from build123d import *

# Parameters (mm, degrees)
SKETCH1_W                  = 10
SKETCH1_H                  = 7
CUT_EXTRUDE1_DEPTH         = 25.841675415
CUT_EXTRUDE2_DEPTH         = 25.841675415
CUT_EXTRUDE3_DEPTH         = 25.841675415
CUT_EXTRUDE4_DEPTH         = 25.841675415
CUT_EXTRUDE5_DEPTH         = 25.841675415
CUT_EXTRUDE6_DEPTH         = 25.841675415
CUT_EXTRUDE7_DEPTH         = 25.841675415
CUT_EXTRUDE8_DEPTH         = 25.841675415
CUT_EXTRUDE9_DEPTH         = 25.73038126
CUT_EXTRUDE10_DEPTH        = 25.73038126
CUT_EXTRUDE11_DEPTH        = 25.73038126
CUT_EXTRUDE12_DEPTH        = 25.590210189
SKETCH14_W                 = 30.0000508
SKETCH14_H                 = 2.5
F_0_8_0_8_DIAMETER_HOLE1_D = 0.8
BOSS_EXTRUDE1_START        = -40.0000508
SKETCH17_R                 = 0.4
BOSS_EXTRUDE1_DEPTH        = 40.0000508
SKETCH18_W                 = 1.5
SKETCH18_H                 = 1.5
CHAMFER1_SIZE              = 0.5
CUT_EXTRUDE13_REACH        = 34.638
CUT_EXTRUDE13_END_RADIUS   = 2
CUT_EXTRUDE13_START        = 5
FILLET1_R                  = 0.5


# Read off the part's stored shape, not the designer's step: Dome1
with BuildPart() as part:
    # Sketch1 → Revolve1 (revolve)
    with BuildSketch(Plane(origin=(0, 0, -7.196357143), x_dir=(-1, 0, 0), z_dir=(0, 0, -1)), mode=Mode.PRIVATE) as revolve1_sk:
        with Locations((-14.77870785, 14.264354232)):
            Rectangle(SKETCH1_W, SKETCH1_H)
    revolve(revolve1_sk.sketch.rotate(Axis((19.77870785, 10.764354232, -7.196357143), (-1, 0, 0)), 270), axis=Axis((19.77870785, 10.764354232, -7.196357143), (-1, 0, 0)))

    # Sketch2 → Cut-Extrude1 (cut, through all)
    with BuildSketch(Plane.ZY.offset(-9.77870785)):
        with BuildLine():
            ThreePointArc((-0.481894482, 12.743240579), (-1.134179317, 14.264354232), (-2.125359964, 15.589806295))
            ThreePointArc((-2.125359964, 15.589806295), (-2.500220073, 14.433413298), (-3.393627672, 13.609042188))
            ThreePointArc((-3.393627672, 13.609042188), (-3.083602501, 13.138854232), (-2.831420372, 12.635270579))
            ThreePointArc((-2.831420372, 12.635270579), (-1.670790249, 12.996798701), (-0.481894482, 12.743240579))
        make_face()
    extrude(amount=-CUT_EXTRUDE1_DEPTH, mode=Mode.SUBTRACT)

    # Sketch3 → Cut-Extrude2 (cut, through all)
    with BuildSketch(Plane.ZY.offset(-9.77870785)):
        with BuildLine():
            ThreePointArc((-0.392018732, 9.12088875), (-0.196357143, 10.764354232), (-0.392018732, 12.407819713))
            ThreePointArc((-0.392018732, 12.407819713), (-1.294853608, 11.593784056), (-2.480752839, 11.326561532))
            ThreePointArc((-2.480752839, 11.326561532), (-2.447357143, 10.764354232), (-2.480752839, 10.202146931))
            ThreePointArc((-2.480752839, 10.202146931), (-1.294853608, 9.934924408), (-0.392018732, 9.12088875))
        make_face()
    extrude(amount=-CUT_EXTRUDE2_DEPTH, mode=Mode.SUBTRACT)

    # Sketch4 → Cut-Extrude3 (cut, through all)
    with BuildSketch(Plane.ZY.offset(-9.77870785)):
        with BuildLine():
            ThreePointArc((-2.125359964, 5.938902169), (-1.134179317, 7.264354232), (-0.481894482, 8.785467884))
            ThreePointArc((-0.481894482, 8.785467884), (-1.670790249, 8.531909762), (-2.831420372, 8.893437884))
            ThreePointArc((-2.831420372, 8.893437884), (-3.083602501, 8.389854232), (-3.393627672, 7.919666275))
            ThreePointArc((-3.393627672, 7.919666275), (-2.500220073, 7.095295166), (-2.125359964, 5.938902169))
        make_face()
    extrude(amount=-CUT_EXTRUDE3_DEPTH, mode=Mode.SUBTRACT)

    # Sketch5 → Cut-Extrude4 (cut, through all)
    with BuildSketch(Plane.ZY.offset(-9.77870785)):
        with BuildLine():
            ThreePointArc((-5.217470795, 4.049891571), (-3.696357143, 4.702176405), (-2.37090508, 5.693357053))
            ThreePointArc((-2.37090508, 5.693357053), (-3.527298077, 6.068217161), (-4.351669187, 6.96162476))
            ThreePointArc((-4.351669187, 6.96162476), (-4.821857143, 6.651599589), (-5.325440796, 6.39941746))
            ThreePointArc((-5.325440796, 6.39941746), (-4.963912674, 5.238787337), (-5.217470795, 4.049891571))
        make_face()
    extrude(amount=-CUT_EXTRUDE4_DEPTH, mode=Mode.SUBTRACT)

    # Sketch6 → Cut-Extrude5 (cut, through all)
    with BuildSketch(Plane.ZY.offset(-9.77870785)):
        with BuildLine():
            ThreePointArc((-8.839822625, 3.960015821), (-7.196357143, 3.764354232), (-5.552891661, 3.960015821))
            ThreePointArc((-5.552891661, 3.960015821), (-6.366927319, 4.862850696), (-6.634149843, 6.048749928))
            ThreePointArc((-6.634149843, 6.048749928), (-7.196357143, 6.015354232), (-7.758564444, 6.048749928))
            ThreePointArc((-7.758564444, 6.048749928), (-8.025786967, 4.862850696), (-8.839822625, 3.960015821))
        make_face()
    extrude(amount=-CUT_EXTRUDE5_DEPTH, mode=Mode.SUBTRACT)

    # Sketch7 → Cut-Extrude6 (cut, through all)
    with BuildSketch(Plane.ZY.offset(-9.77870785)):
        with BuildLine():
            ThreePointArc((-12.021809206, 5.693357053), (-10.696357143, 4.702176405), (-9.175243491, 4.049891571))
            ThreePointArc((-9.175243491, 4.049891571), (-9.428801613, 5.238787337), (-9.067273491, 6.39941746))
            ThreePointArc((-9.067273491, 6.39941746), (-9.570857143, 6.651599589), (-10.0410451, 6.96162476))
            ThreePointArc((-10.0410451, 6.96162476), (-10.865416209, 6.068217161), (-12.021809206, 5.693357053))
        make_face()
    extrude(amount=-CUT_EXTRUDE6_DEPTH, mode=Mode.SUBTRACT)

    # Sketch8 → Cut-Extrude7 (cut, through all)
    with BuildSketch(Plane.ZY.offset(-9.77870785)):
        with BuildLine():
            ThreePointArc((-13.910819804, 8.785467884), (-13.25853497, 7.264354232), (-12.267354322, 5.938902169))
            ThreePointArc((-12.267354322, 5.938902169), (-11.892494213, 7.095295166), (-10.999086614, 7.919666275))
            ThreePointArc((-10.999086614, 7.919666275), (-11.309111786, 8.389854232), (-11.561293915, 8.893437884))
            ThreePointArc((-11.561293915, 8.893437884), (-12.721924037, 8.531909762), (-13.910819804, 8.785467884))
        make_face()
    extrude(amount=-CUT_EXTRUDE7_DEPTH, mode=Mode.SUBTRACT)

    # Sketch9 → Cut-Extrude8 (cut, through all)
    with BuildSketch(Plane.ZY.offset(-9.77870785)):
        with BuildLine():
            ThreePointArc((-14.000695554, 12.407819713), (-14.196357143, 10.764354232), (-14.000695554, 9.12088875))
            ThreePointArc((-14.000695554, 9.12088875), (-13.097860679, 9.934924408), (-11.911961447, 10.202146931))
            ThreePointArc((-11.911961447, 10.202146931), (-11.945357143, 10.764354232), (-11.911961447, 11.326561532))
            ThreePointArc((-11.911961447, 11.326561532), (-13.097860679, 11.593784056), (-14.000695554, 12.407819713))
        make_face()
    extrude(amount=-CUT_EXTRUDE8_DEPTH, mode=Mode.SUBTRACT)

    # Sketch10 → Cut-Extrude9 (cut, through all)
    with BuildSketch(Plane.ZY.offset(-9.77870785)):
        with BuildLine():
            ThreePointArc((-12.267354322, 15.589806295), (-13.25853497, 14.264354232), (-13.910819804, 12.743240579))
            ThreePointArc((-13.910819804, 12.743240579), (-12.721924037, 12.996798701), (-11.561293915, 12.635270579))
            ThreePointArc((-11.561293915, 12.635270579), (-11.309111786, 13.138854232), (-10.999086614, 13.609042188))
            ThreePointArc((-10.999086614, 13.609042188), (-11.892494213, 14.433413298), (-12.267354322, 15.589806295))
        make_face()
    extrude(amount=-CUT_EXTRUDE9_DEPTH, mode=Mode.SUBTRACT)

    # Sketch11 → Cut-Extrude10 (cut, through all)
    with BuildSketch(Plane.ZY.offset(-9.77870785)):
        with BuildLine():
            ThreePointArc((-9.175243491, 17.478816892), (-10.696357143, 16.826532058), (-12.021809206, 15.83535141))
            ThreePointArc((-12.021809206, 15.83535141), (-10.865416209, 15.460491302), (-10.0410451, 14.567083703))
            ThreePointArc((-10.0410451, 14.567083703), (-9.570857143, 14.877108874), (-9.067273491, 15.129291003))
            ThreePointArc((-9.067273491, 15.129291003), (-9.428801613, 16.289921126), (-9.175243491, 17.478816892))
        make_face()
    extrude(amount=-CUT_EXTRUDE10_DEPTH, mode=Mode.SUBTRACT)

    # Sketch12 → Cut-Extrude11 (cut, through all)
    with BuildSketch(Plane.ZY.offset(-9.77870785)):
        with BuildLine():
            ThreePointArc((-5.552891661, 17.568692642), (-7.196357143, 17.764354232), (-8.839822625, 17.568692642))
            ThreePointArc((-8.839822625, 17.568692642), (-8.025786967, 16.665857767), (-7.758564444, 15.479958536))
            ThreePointArc((-7.758564444, 15.479958536), (-7.196357143, 15.513354232), (-6.634149843, 15.479958536))
            ThreePointArc((-6.634149843, 15.479958536), (-6.366927319, 16.665857767), (-5.552891661, 17.568692642))
        make_face()
    extrude(amount=-CUT_EXTRUDE11_DEPTH, mode=Mode.SUBTRACT)

    # Sketch13 → Cut-Extrude12 (cut, through all)
    with BuildSketch(Plane.ZY.offset(-9.77870785)):
        with BuildLine():
            ThreePointArc((-2.37090508, 15.83535141), (-3.696357143, 16.826532058), (-5.217470795, 17.478816892))
            ThreePointArc((-5.217470795, 17.478816892), (-4.963912674, 16.289921126), (-5.325440796, 15.129291003))
            ThreePointArc((-5.325440796, 15.129291003), (-4.821857143, 14.877108874), (-4.351669187, 14.567083703))
            ThreePointArc((-4.351669187, 14.567083703), (-3.527298077, 15.460491302), (-2.37090508, 15.83535141))
        make_face()
    extrude(amount=-CUT_EXTRUDE12_DEPTH, mode=Mode.SUBTRACT)

    # Sketch14 → Revolve2 (revolve)
    with BuildSketch(Plane.XY.offset(-7.196357143), mode=Mode.PRIVATE) as revolve2_sk:
        with Locations((-5.22131755, 12.014354232)):
            Rectangle(SKETCH14_W, SKETCH14_H)
    revolve(revolve2_sk.sketch.rotate(Axis((-20.22134295, 10.764354232, -7.196357143), (1, 0, 0)), 270), axis=Axis((-20.22134295, 10.764354232, -7.196357143), (1, 0, 0)))

    # Ø0.8 (0.8) Diameter Hole1 (through all)
    with Locations(Plane(origin=(19.77870785, 0, 0), x_dir=(0, 0, -1), z_dir=(1, 0, 0))):
        with Locations((7.196357143, 10.764354232)):
            Hole(F_0_8_0_8_DIAMETER_HOLE1_D / 2)

    # Sketch17 → Boss-Extrude1 (add)
    with BuildSketch(Plane(origin=(19.77870785, 0, 0), x_dir=(0, 0, -1), z_dir=(1, 0, 0)).offset(BOSS_EXTRUDE1_START)):
        with Locations((7.196357143, 10.764354232)):
            Circle(SKETCH17_R)
    extrude(amount=BOSS_EXTRUDE1_DEPTH)

    # Sketch18 → Revolve3 (revolve)
    with BuildSketch(Plane.XY.offset(-7.196357143), mode=Mode.PRIVATE) as revolve3_sk:
        with Locations((-9.47134295, 14.014354232)):
            Rectangle(SKETCH18_W, SKETCH18_H)
    revolve(revolve3_sk.sketch.rotate(Axis((-20.22134295, 10.764354232, -7.196357143), (1, 0, 0)), 90), axis=Axis((-20.22134295, 10.764354232, -7.196357143), (1, 0, 0)))

    # Chamfer1
    chamfer1_edges = [part.edges().sort_by_distance(p)[0] for p in [
        (-20.22134295, 10.764354232, -4.696357143),
    ]]
    chamfer(chamfer1_edges, length=CHAMFER1_SIZE)

    # Cut-Extrude13: up to this cylinder (the profile starts outside it)
    cut_extrude13_end = Plane(origin=(-15.221343, 10.764354232, -7.196357143), z_dir=(1, 0, 0)) * Cylinder(CUT_EXTRUDE13_END_RADIUS, 74.276, mode=Mode.PRIVATE)
    # Sketch20 → Cut-Extrude13 (cut, up to the surface)
    with BuildSketch(Plane.XY.offset(-7.196357143).offset(CUT_EXTRUDE13_START), mode=Mode.PRIVATE) as cut_extrude13_sk1:
        with BuildLine():
            Line((-12.72134295, 9.882388481), (-17.72134295, 9.882388481))
            ThreePointArc((-17.72134295, 9.882388481), (-18.47134295, 10.632388481), (-17.72134295, 11.382388481))
            Line((-17.72134295, 11.382388481), (-12.72134295, 11.382388481))
            ThreePointArc((-12.72134295, 11.382388481), (-11.97134295, 10.632388481), (-12.72134295, 9.882388481))
        make_face()
    cut_extrude13_tool1 = extrude(cut_extrude13_sk1.sketch, amount=-CUT_EXTRUDE13_REACH, mode=Mode.PRIVATE) - cut_extrude13_end
    add(cut_extrude13_tool1.solids().sort_by_distance((-15.221343, 10.632388, -2.196357))[0], mode=Mode.SUBTRACT)

    # Dome1 outline → Dome1 (revolve, cut)
    with BuildSketch(Plane(origin=(0, 10.764354232, -7.196357143), x_dir=(0, 1, 0), z_dir=(0, 0, -1))):
        with BuildLine():
            Line((0, 19.778707854), (0, 19.27870785))
            ThreePointArc((0, 19.27870785), (1.891593251, 19.404258523), (3.750000014, 19.778707854))
            Line((3.750000014, 19.778707854), (0, 19.778707854))
        make_face()
    revolve(axis=Axis((0, 10.764354232, -7.196357143), (1, 0, 0)), mode=Mode.SUBTRACT)

    # Fillet1
    fillet1_edges = [part.edges().sort_by_distance(p)[0] for p in [
        (19.778707854, 7.014354218, -7.196357143),
    ]]
    fillet(fillet1_edges, radius=FILLET1_R)


solid = part.part
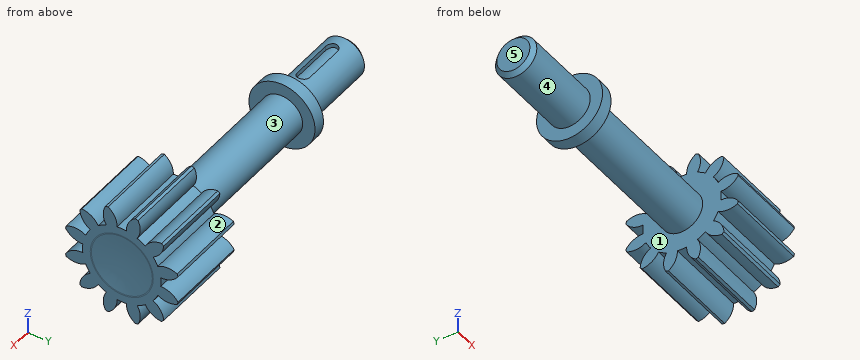
Source: CAD feature listing. Evaluate the final solid. Frame: model axes, mm. Face numbers are marked on the shaded views. A direction names the side the tool comes from. Round coordinates to 2 decimals unless told otherwise and drop trailing zeros. Loops run counter-clockwise (first coordinate to the right, second up) from the corner with the lowest first, then second, coordinate; pieces in that order, holes last. Notation, with made-up numbers: (15, 58) -> (33, 58) arc R15 ccw to (33, 63) -> close; hole circle Ø9 at (9.25, 23.25). An arc over 180 degrees is marked (long way). Answer as a JSON object with one key per item and string values. Group by question number.
Q1. Section query B-B (y = 16.5). Output: boundary loops of the cut face in (x, z), plus the area to 3 significant figures.
Q2. Access query for the marked faces 4 and 5. Directions: +Z, -Z, +X, -X, +Y, -Y. A direction counts if a zero-diameter tool reaches every point of the face in a straight line with its end or side. Return the directions, or none.
Q3. Section query C-C (x = 1). Output: boundary loops of the cut face in (y, z).
Q4. Mould query, pull axis Y, two halves, no side actions, for the marked faces 1, 2 and 3. Classes: pulls with the +Y half, pulls with the -Y half, needs draft (parallel to the pull), parting line crosses it, or undercut.
Q5. Ray query, line 1 (X direction, y = 14.25, z = -8.75); line 2 (X direction, y = 5, z = -8.5); line 3 (X direction, y = 8.75, z = -9.5). Return the intervals inside material, ascending. Write a range as from..to.
Q6. Section query A-A (y = 5.25). Output: boundary loops of the cut face in (x, z).
Q7. Contact query for flat-ended pins moving along their axis: P1, Ø3, axis at x = 7, y = 6, coming from the +Z side; P2, Ø3, axis at x = -3.5, z = -10, coming from the +Y side; P3, Ø4, axis at y = 10, z = -7, coming from the +X side; P4, Ø6, axis at x = -15.5, z = -10, coming from the -Y side. Output: stop coordinate, or through.
Completed:
{
 "1": {"outline": "(9.78, -9.43) -> (19.78, -9.43) -> (19.78, -7.95) -> (9.78, -7.95) -> close; (9.78, -6.44) -> (19.78, -6.44) -> (19.78, -4.96) -> (9.78, -4.96) -> close", "area": "29.6 mm²"},
 "2": {"face 4": "-X", "face 5": "+Z, -Z, -X, +Y, -Y"},
 "3": {"outline": "circle Ø5 at (10.76, -7.2)"},
 "4": {"face 1": "needs draft", "face 2": "undercut", "face 3": "parting line crosses it"},
 "5": {"line 1": "-10.22..-8.72, 9.78..19.78", "line 2": "9.78..19.78", "line 3": "-10.22..-8.72, 9.78..19.61"},
 "6": {"outline": "(9.78, -9.43) -> (19.78, -9.43) -> (19.78, -7.87) -> (9.78, -7.87) -> close; (9.78, -6.53) -> (19.78, -6.53) -> (19.78, -4.96) -> (9.78, -4.96) -> close"},
 "7": {"P1": "through", "P2": "y = 12.9", "P3": "x = 19.55", "P4": "y = 8.26"}
}
